Design review of the part built by this model. Coordinates are the model's own, in mm. Face numbers are marked on the shaded views. A direction names the side the tool comes from. Coordinates: 2 decimals unless noted, no trailing zeros. Order: outer loops, then holes, each group sorted by start corner. A loop starts at its lowest first (then second) coordinate and runs counter-clockwise, first axis right, second up. Notation, with made-up numbers: M 80.25,13.5 L 135.25,13.5 A23 cw 135.25,49.5 Z; hole C 17.25,53.25 d3. An arc over 180 degrees is marked long. Answer as a JSON object with one key per item and string values.
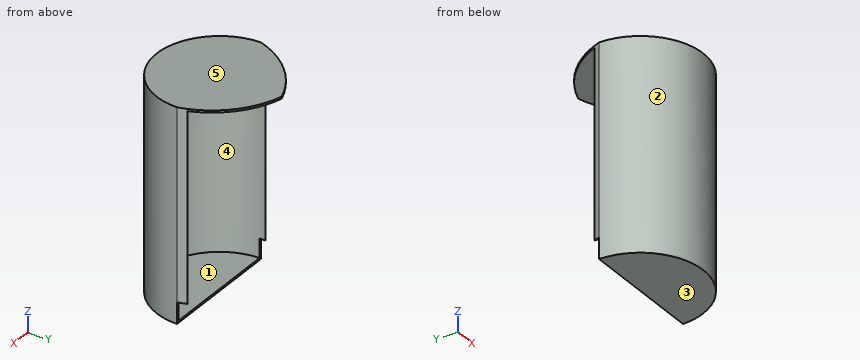
from build123d import *

# Parameters (mm, degrees)
F1_DEPTH = 254
F2_T     = -2.54
F4_DEPTH = 25.4


with BuildPart() as f1:
    # F0 (on Top) → F1 (new body)
    with BuildSketch(Plane.XY):
        with BuildLine():
            ThreePointArc((-0.185259, 75.771093), (-46.959517, 46.774258), (-75.956352, 0))
            ThreePointArc((-75.956352, 0), (-0.185259, -75.035728), (75.585835, 0))
            ThreePointArc((75.585835, 0), (48.21746, 48.402718), (-0.185259, 75.771093))
        make_face()
    extrude(amount=F1_DEPTH)

    # F2
    f2_openings = [f1.faces().sort_by_distance(p)[0] for p in [
        (-46.959517, 46.774258, 127),
        (48.21746, 48.402718, 127),
    ]]
    offset(amount=F2_T, openings=f2_openings)

    # F3 (on face) → F4 (cut)
    with BuildSketch(Plane(origin=(0, 0, 0), x_dir=(1, 0, 0), z_dir=(0, 0, -1))):
        with BuildLine():
            ThreePointArc((-0.185259, -75.771093), (48.21746, -48.402718), (75.585835, 0))
            Line((75.585835, 0), (0, 0))
            Line((0, 0), (-0.185259, -75.771093))
        make_face()
        with BuildLine():
            Line((-0.185259, -75.771093), (0, 0))
            Line((0, 0), (-75.956352, 0))
            ThreePointArc((-75.956352, 0), (-46.959517, -46.774258), (-0.185259, -75.771093))
        make_face()
    extrude(amount=-F4_DEPTH, mode=Mode.SUBTRACT)


solid = f1.part
1) Add section D-D (y = -16). State the section outline as (x, z) points, and give its area (3 significant figures).
Taken from the geometry:
{"outline": "M -74.09,0 L 73.72,0 L 73.72,254 L -74.09,254 Z; hole M -71.48,2.54 L 71.11,2.54 L 71.11,251.46 L -71.48,251.46 Z", "area": "2,050 mm2"}
2) Insertion check: pin 1 Ø6 at (y, z) = (-8, 118) entering from +X; pin 2 Ø3 at (y, z) = (-22.5, 196) entering from -X; pin 3 Ø4 at (x, y) = (46, 6) entering from -Z. Each pin has a flat end and moves straight along its axis. Give the tip position at first contact, or say it passes through.
Taken from the geometry:
{"pin 1": "stops at x = 75.37", "pin 2": "stops at x = -72.77", "pin 3": "stops at z = 251.46"}
3) To check wall thickness, follow L1, parallel to Z at x = 30, y = -31; L2, parallel to Z at x = 41, y = 33; L3, parallel to Y at x = -1.5, z = 105.5. State the ranges of each line that lie inside material, in increasing order.
Taken from the geometry:
{"L1": "z = 0 to 2.54, 251.46 to 254", "L2": "z = 251.46 to 254", "L3": "y = -75.02 to -72.48"}
4) Add section B-B (x = 14). State the section outline as (y, z) points, and give its area (3 significant figures).
Taken from the geometry:
{"outline": "M -73.7,0 L 0,0 L 0,2.54 L -71.11,2.54 L -71.11,251.46 L 71.14,251.46 L 71.14,254 L -73.7,254 Z", "area": "1,200 mm2"}
5) Tool access review of the marked faces 4 and 5: name each direction out of +Z, -Z, +X, -X, +Y, -Y from which nothing blocks a thin tool from reaching the whole face with its end or side.
Taken from the geometry:
{"face 4": "none", "face 5": "+Z, +X, -X, +Y, -Y"}
6) Mouldability with a two-part tool opening along X and no side actions: class the marked faces 1, 2 and 3 as released by +X, released by -X, zero draft, split by the parting line, or undercut.
Taken from the geometry:
{"face 1": "undercut", "face 2": "split by the parting line", "face 3": "zero draft"}
7) Add section A-A (y = -50.5). State the section outline as (x, z) points.
Taken from the geometry:
{"outline": "M -56.01,0 L 55.64,0 L 55.64,254 L -56.01,254 Z; hole M -52.51,2.54 L 52.14,2.54 L 52.14,251.46 L -52.51,251.46 Z"}
